Part model, mm, in its own coordinate system. A direction names the side the tool comes from. Coordinates: 2 decimals unless noted, no trailing zeros. Loops run counter-clockwise (first coordinate to the right, second up) from the corner with the lowest first, then second, coordinate; pieces in that order, holes last. Notation, with made-up numbers: M 71,-40 L 77,-40 A9 ccw 77,-31 Z; hole C -1.5,26.25 d8. An arc over 180 degrees is marked long. Use a Markdown table: item, result. Add a question column.
1) Tool access for faces 1 (the flat face through (-19, 53, 0)), 2 (the cylindrical face through (-67.06, 34.88, 0.06)), 3 (the flat face through (-36, 58.922, 0)): list every direction of +Z, -Z, +X, -X, +Y, -Y with a clear straight run to the whole face (end or side of a thin tool).
2) Pin check, flat tips, straight feed: pin 1 Ø6 at (x, y) = (-42.5, 42.5) entering from -Z; pin 2 Ø2.5 at (x, z) = (-55, -0.5) entering from +Y; pin 3 Ø1.7 at (x, z) = (-72, 1.5) entering from -Y; pin 4 Ø1.5 at (y, z) = (55, 1) entering from +X. Stop position of each tip, or through.
3) Pull direction Y, two halves, no side cores. Call faces 4 (the flat face through (-60.02, 66, 0)), 5 (the flat face through (-49.812, 37, 0)), 6 (the cylindrical face through (-79.817, 63.238, 0.061)), 7 (the cylindrical face through (-46, 42, 0)): released by +Y, released by -Y, zero draft, split by the parting line, or undercut.
4) Band-saw the part on C-C (y = 11.5). List the corners of the cut face in (x, z).
5) Band-saw the part on D-D (y = -7). List the corners of the cut face in (x, z).
6) Wall check: probe 1 along Z at (x, y) = (-45.85, 45); probe 2 along Y at (x, z) = (-58, 2); probe 3 along Y at (x, z) = (-67.5, 2.25). Give the ranges that are in metal, low to high. Write a range as from..to.
7) Band-saw the part on A-A (x = -57.5). List the corners of the cut face in (y, z), plus the area to 3 significant figures.
8) Band-saw the part on B-B (z = 1.5). State how many separate pieces and enclosed holes the cut face has, plus the area to 3 significant figures.
from build123d import *

# Parameters (mm, degrees)
F0_R     = 2.25
F1_DEPTH = 4.330125
F2_W     = 20
F2_H     = 16
F3_DEPTH = 12.5
F4_R     = 3.2
F5_W     = 6.4
F5_H     = 8.66025
F5_R     = 3
F6_DEPTH = 3.2
F8_DEPTH = 2.5
F9_R     = 1.6
F10_R    = 5


# Not quite as in the source:
# - ends of sketch curves that miss each other by under 0.0002 mm in the source are joined


with BuildPart() as f1:
    # F0 (on Top) → F1 (new body, symmetric)
    with BuildSketch(Plane.XY):
        with BuildLine():
            Line((20, -24.8214285714), (0, 27.4853587511))
            Line((0, 27.4853587511), (-3.829193786, 37.5))
            Line((-3.829193786, 37.5), (-12.6123318144, 37.5))
            Line((-12.6123318144, 37.5), (-25.6123318144, 37.5))
            Line((-25.6123318144, 37.5), (-25.6123318144, 38.8834841531))
            Line((-25.6123318144, 38.8834841531), (-30.6123318144, 38.8834841531))
            Line((-30.6123318144, 38.8834841531), (-30.6123318144, 34.3834841531))
            Line((-30.6123318144, 34.3834841531), (-44.1123318144, 34.3834841531))
            Line((-44.1123318144, 34.3834841531), (-44.1123318144, 41.8))
            Line((-44.1123318144, 41.8), (-47.3123318144, 41.8))
            Line((-47.3123318144, 41.8), (-47.3123318144, 34.3834841531))
            Line((-47.3123318144, 34.3834841531), (-64.3336698413, 34.3834841531))
            Line((-64.3336698413, 34.3834841531), (-64.3336698413, 36.2610286334))
            ThreePointArc((-64.3336698413, 36.2610286334), (-67.1028911134, 34.8644323695), (-70.1668349206, 34.3834792274))
            Line((-70.1668349206, 34.3834792274), (-76, 34.3834841531))
            ThreePointArc((-76, 34.3834841531), (-83.0710678119, 37.3124163412), (-86, 44.3834841531))
            Line((-86, 44.3834841531), (-86, 45.6165158469))
            ThreePointArc((-86, 45.6165158469), (-83.0710678119, 52.6875836588), (-76, 55.6165158469))
            Line((-76, 55.6165158469), (-70.1668349206, 55.6165158469))
            ThreePointArc((-70.1668349206, 55.6165158469), (-67.1028911134, 55.1355676305), (-64.3336698413, 53.7389713666))
            Line((-64.3336698413, 53.7389713666), (-64.3336698413, 55.6165158469))
            Line((-64.3336698413, 55.6165158469), (-47.3123318144, 55.6165158469))
            Line((-47.3123318144, 55.6165158469), (-47.3123318144, 48.2))
            Line((-47.3123318144, 48.2), (-44.1123318144, 48.2))
            Line((-44.1123318144, 48.2), (-44.1123318144, 55.6165158469))
            Line((-44.1123318144, 55.6165158469), (-30.6123318144, 55.6165158469))
            Line((-30.6123318144, 55.6165158469), (-30.6123318144, 51.1165158469))
            Line((-30.6123318144, 51.1165158469), (-25.6123318144, 51.1165158469))
            Line((-25.6123318144, 51.1165158469), (-25.6123318144, 52.5))
            Line((-25.6123318144, 52.5), (-12.6123318144, 52.5))
            Line((-12.6123318144, 52.5), (-9.5645871327, 52.5))
            Line((-9.5645871327, 52.5), (-12.0202176002, 58.9223070303))
            Line((-12.0202176002, 58.9223070303), (-60.0202176002, 58.9223070303))
            Line((-60.0202176002, 58.9223070303), (-60.0202176002, 73.9223070303))
            Line((-60.0202176002, 73.9223070303), (-78.0202176002, 73.9223070303))
            Line((-78.0202176002, 73.9223070303), (-78.0202176002, 71.5223070303))
            ThreePointArc((-78.0202176002, 71.5223070303), (-79.8672373555, 63.1277070855), (-85.0671484236, 56.2836063342))
            ThreePointArc((-85.0671484236, 56.2836063342), (-88.7070861713, 51.4927358083), (-90, 45.6165158469))
            Line((-90, 45.6165158469), (-90, 44.3834841531))
            ThreePointArc((-90, 44.3834841531), (-85.8994949366, 34.4839892165), (-76, 30.3834841531))
            Line((-76, 30.3834841531), (-50, 30.3834841531))
            Line((-50, 30.3834841531), (-47.7142857143, 24.405565602))
            ThreePointArc((-47.7142857143, 24.405565602), (-36.0935520375, 19.2134033537), (-41.2857142857, 7.5926696769))
            Line((-41.2857142857, 7.5926696769), (-40.1428571429, 4.6037104013))
            ThreePointArc((-40.1428571429, 4.6037104013), (-27.2309308353, -1.1653587634), (-33, -14.077285071))
            Line((-33, -14.077285071), (-31.8571428571, -17.0662443466))
            ThreePointArc((-31.8571428571, -17.0662443466), (-21.5276018111, -21.6814996784), (-26.1428571429, -32.0110407244))
            Line((-26.1428571429, -32.0110407244), (-25, -35))
            Line((-25, -35), (12.9946266979, -35))
            ThreePointArc((12.9946266979, -35), (19.1727852307, -31.7521003214), (20, -24.8214285714))
        make_face()
        with Locations((-5.1674522335, -15)):
            Circle(F0_R, mode=Mode.SUBTRACT)
        with Locations((-67.5202176002, 66.4223070303)):
            Circle(F0_R, mode=Mode.SUBTRACT)
        with Locations((-23.0245950907, 31.7024886808)):
            Circle(F0_R, mode=Mode.SUBTRACT)
    extrude(amount=F1_DEPTH, both=True)

    # F2 (on Top) → F3 (cut, symmetric)
    with BuildSketch(Plane.XY):
        with Locations((-17.4123318144, 45)):
            Rectangle(F2_W, F2_H)
    extrude(amount=F3_DEPTH, both=True, mode=Mode.SUBTRACT)

    # F4
    f4_edges = [f1.edges().sort_by_distance(p)[0] for p in [
        (-44.112332, 55.616516, 0),
        (-44.112332, 34.383484, 0),
    ]]
    fillet(f4_edges, radius=F4_R)

    # F5 (on face) → F6 (join)
    with BuildSketch(Plane.YZ.offset(-44.1123318144)):
        with Locations((45, 0)):
            Rectangle(F5_W, F5_H)
        with Locations((45, 0)):
            Circle(F5_R, mode=Mode.SUBTRACT)
    extrude(amount=-F6_DEPTH)

    # F7 (on face) → F8 (join)
    with BuildSketch(Plane(origin=(-47.3123318144, 0, 0), x_dir=(0, -1, 0), z_dir=(-1, 0, 0))):
        with BuildLine():
            Line((-48.3911675695, 4.330125), (-55.6165158469, 4.330125))
            Line((-55.6165158469, 4.330125), (-55.6165158469, -4.330125))
            Line((-55.6165158469, -4.330125), (-48.3911675695, -4.330125))
            ThreePointArc((-48.3911675695, -4.330125), (-50.5, 0), (-48.3911675695, 4.330125))
        make_face()
        with BuildLine():
            Line((-34.3834841531, -4.330125), (-34.3834841531, 4.330125))
            Line((-34.3834841531, 4.330125), (-41.6088324305, 4.330125))
            ThreePointArc((-41.6088324305, 4.330125), (-39.5, 0), (-41.6088324305, -4.330125))
            Line((-41.6088324305, -4.330125), (-34.3834841531, -4.330125))
        make_face()
    extrude(amount=F8_DEPTH)

    # F9
    f9_edges = [f1.edges().sort_by_distance(p)[0] for p in [
        (-25, -35, 0),
        (-26.142857, -32.011041, 0),
        (-31.857143, -17.066244, 0),
        (-33, -14.077285, 0),
        (-40.142857, 4.60371, 0),
        (-41.285714, 7.59267, 0),
        (-47.714286, 24.405566, 0),
    ]]
    fillet(f9_edges, radius=F9_R)

    # F10
    f10_edges = [f1.edges().sort_by_distance(p)[0] for p in [
        (-50, 30.383484, 0),
    ]]
    fillet(f10_edges, radius=F10_R)


solid = f1.part
Entries:
| question | item | result |
|---|---|---|
| 1 | face 1 | +Z, -Z, +X |
| 1 | face 2 | +Z, -Z |
| 1 | face 3 | +Z, -Z, +X, +Y |
| 2 | pin 1 | z = -4.33 |
| 2 | pin 2 | y = 58.92 |
| 2 | pin 3 | y = 30.38 |
| 2 | pin 4 | x = -10.23 |
| 3 | face 4 | zero draft |
| 3 | face 5 | undercut |
| 3 | face 6 | released by +Y |
| 3 | face 7 | undercut |
| 4 | outline | M -36.71,-4.33 L 6.11,-4.33 L 6.11,4.33 L -36.71,4.33 Z |
| 5 | outline | M -26.83,-4.33 L 13.19,-4.33 L 13.19,4.33 L -26.83,4.33 Z |
| 6 | probe 1 | -4.33..-3, 3..4.33 |
| 6 | probe 2 | 30.38..34.38, 55.62..58.92 |
| 6 | probe 3 | 30.38..34.75, 55.25..64.17, 68.67..73.92 |
| 7 | outline | M 30.38,-4.33 L 34.38,-4.33 L 34.38,4.33 L 30.38,4.33 Z; M 55.62,-4.33 L 58.92,-4.33 L 58.92,4.33 L 55.62,4.33 Z |
| 7 | area | 63.3 mm2 |
| 8 | separate pieces | 1 |
| 8 | enclosed holes | 3 |
| 8 | area | 3,920 mm2 |
